Build history of the part. All positions in model axes, mm. Round coordinates to 2 decimals unless told otherwise and drop trailing zeros. Write each loop counter-clockwise with the first axis right and the second up, starting at its lowest first coordinate (ties: lowest second). Pieces come first, ordered by that corner, then holes.
from build123d import *

# Parameters (mm, degrees)
SKETCH_1_R      = 2
SKETCH_1_W      = 1.855595784
SKETCH_1_H      = 1.9
EXTRUDE_1_DEPTH = 2.5
SKETCH_2_R      = 4.5
EXTRUDE_2_DEPTH = 2
FILLET_2_R      = 0.5
SKETCH_4_W      = 1.855595784
SKETCH_4_H      = 1.9
EXTRUDE_3_DEPTH = 0.5


with BuildPart() as part:
    # 草图1 → 凸台-拉伸1 (new body)
    with BuildSketch(Plane(origin=(0, 0, 0), x_dir=(1, 0, 0), z_dir=(0, 1, 0))):
        with Locations(Location((0, 0, 0), (0, 0, 270))):
            Circle(SKETCH_1_R)
        Rectangle(SKETCH_1_W, SKETCH_1_H, mode=Mode.SUBTRACT)
    extrude(amount=EXTRUDE_1_DEPTH)

    # 草图2 → 凸台-拉伸2 (add)
    with BuildSketch(Plane(origin=(0, 2.5, 0), x_dir=(1, 0, 0), z_dir=(0, 1, 0))):
        with Locations(Location((0, 0, 0), (0, 0, 270))):
            Circle(SKETCH_2_R)
    extrude(amount=EXTRUDE_2_DEPTH)

    # 草图3 → 切除-旋转6 (revolve, cut)
    with BuildSketch(Plane.XY, mode=Mode.PRIVATE) as cut_revolve_6_sk:
        with BuildLine():
            Line((-5.348495513, 4.5), (0, 4.5))
            Line((0, 4.5), (0, 3.454223495))
            ThreePointArc((0, 3.454223495), (-2.724887739, 3.718119778), (-5.348495513, 4.5))
        make_face()
    revolve(cut_revolve_6_sk.sketch.rotate(Axis((0, 4.5, 0), (0, -1, 0)), 270), axis=Axis((0, 4.5, 0), (0, -1, 0)), mode=Mode.SUBTRACT)

    # 圆角2
    fillet_2_edges = [part.edges().sort_by_distance(p)[0] for p in [
        (0, 2.5, -4.5),
        (0, 4.186113011, -4.5),
        (0, 2.5, -2),
    ]]
    fillet(fillet_2_edges, radius=FILLET_2_R)

    # 草图4 → 凸台-拉伸3 (add)
    with BuildSketch(Plane.XZ.offset(-2.5)):
        Rectangle(SKETCH_4_W, SKETCH_4_H)
    extrude(amount=EXTRUDE_3_DEPTH)


solid = part.part
1) Wall check: L1, parallel to X at y = 0.6, z = 0.75; L2, parallel to Z at x = 0.5, y = 0.75; L3, parallel to X at y = 3.05, z = 4. Give the ranges that are in metal, low to high.
Results:
L1: x = -1.85 to -0.93, 0.93 to 1.85
L2: z = -1.94 to -0.95, 0.95 to 1.94
L3: x = -2.06 to 2.06
2) Mould opens along Z. For faces 1 (the flat face through (0, 1, -0.95)), 2 (the flat face through (0, 0, 1.3)), 3 (the cylindrical face through (1.352, 3.251, 4.292)) say: released by +Z, released by -Z, zero draft, split by the parting line, or undercut.
Results:
face 1: undercut
face 2: zero draft
face 3: split by the parting line
3) Slice it at A-A (y = 0.9). Write the cut outline in (x, z), plus the area to 3 significant figures.
Results:
outline: circle Ø4 at (0, 0); hole (-0.93, -0.95) - (0.93, -0.95) - (0.93, 0.95) - (-0.93, 0.95) - close
area: 9.04 mm2
4) Pin check, flat tips, straight feed: pin 1 Ø0.9 at (x, z) = (0, 0) entering from -Y; pin 2 Ø1 at (x, y) = (1, 1.5) entering from -Z; pin 3 Ø1.5 at (y, z) = (1.5, 0.5) entering from +X. Stop position of each tip, or through.
Results:
pin 1: stops at y = 2
pin 2: stops at z = -1.94
pin 3: stops at x = 2.03
